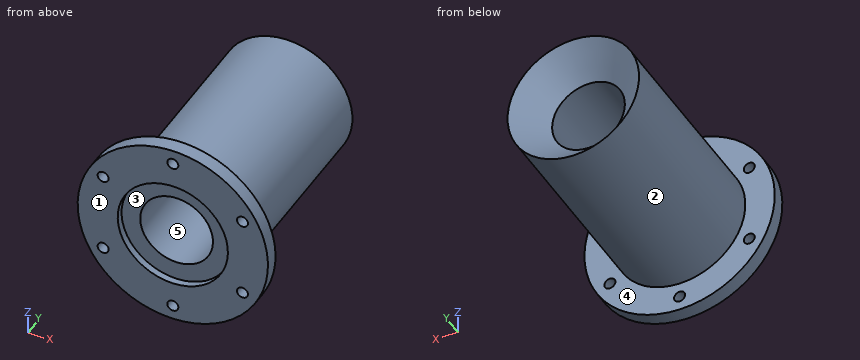
```python
from build123d import *

# Parameters (mm, degrees)
SKETCH_2_R          = 1.5
CUT_EXTRUDE_1_DEPTH = 10


with BuildPart() as part:
    # Эскиз1 → Повернуть1 (revolve)
    with BuildSketch(Plane(origin=(0, 0, 0), x_dir=(0, 0, -1), z_dir=(1, 0, 0))):
        Polygon((9.9, 52), (9.9, 2), (15, 2), (15, 0), (25.9, 0), (25.9, 4), (17.9, 4), (17.9, 60), align=None)
    revolve(axis=Axis((0, 0, 0), (0, 1, 0)))

    # Эскиз2 → Вырез-Вытянуть1 (cut)
    with BuildSketch(Plane(origin=(0, 4, 0), x_dir=(1, 0, 0), z_dir=(0, 1, 0))):
        with Locations(Location((0, 21.9, 0), (0, 0, 270))):
            Circle(SKETCH_2_R)
        with Locations(Location((18.965956343, 10.95, 0), (0, 0, 270))):
            Circle(SKETCH_2_R)
        with Locations(Location((18.965956343, -10.95, 0), (0, 0, 270))):
            Circle(SKETCH_2_R)
        with Locations(Location((0, -21.9, 0), (0, 0, 270))):
            Circle(SKETCH_2_R)
        with Locations(Location((-18.965956343, -10.95, 0), (0, 0, 270))):
            Circle(SKETCH_2_R)
        with Locations(Location((-18.965956343, 10.95, 0), (0, 0, 270))):
            Circle(SKETCH_2_R)
    extrude(amount=-CUT_EXTRUDE_1_DEPTH, mode=Mode.SUBTRACT)


solid = part.part
```
The model under review builds one solid part; all positions refer to its coordinate system, in mm. Face numbers are marked on the shaded views. A direction names the side the tool comes from. Round coordinates to 2 decimals unless told otherwise and drop trailing zeros. Write each loop counter-clockwise with the first axis right and the second up, starting at its lowest first coordinate (ties: lowest second). Pieces come first, ordered by that corner, then holes. Notation, with made-up numbers: M 29.5,-35 L 70.5,-35 A24 ccw 70.5,-25 Z; hole C 20.25,24 d2. An arc over 180 degrees is marked long. Use CSV: the item, a comma, the result in double quotes. Start each with the question number.
(1) For line 1 along Y through (x, z) = (15, 12.5); line 2 along X through (y, z) = (21, 0); line 3 along X through (y, z) = (1.4, 21.9), list the stretches that pass through material, from the lowest coordinate up.
(2) We need section A-A, the plane z = 0. State the section outline as (x, y) points, then the cut area to 3 significant figures.
(3) We need section D-D, the plane z = 21.9. State the section outline as (x, y) points, then the cut area to 3 significant figures.
(4) We need section C-C, the plane y = 53.5. State the section outline as (x, z) points, then the cut area to 3 significant figures.
(5) The part is to be moulded in two halves that separate along Z. For the marked faces 1, 2 and 3, say which applies: +Z half, -Z half, draft (parallel to the pull), parting line (faces both ways), or undercut.
(6) Tool access review of the marked faces 4 and 5: name each direction out of +Z, -Z, +X, -X, +Y, -Y from which nothing blocks a thin tool from reaching the whole face with its end or side.
(7) We need section B-B, the plane x = 0. State the section outline as (y, z) points, then the cut area to 3 significant figures.
(8) Clearance check with flat-ended pins moving along their axes: P1, Ø6, axis at x = -12.5, z = -16, coming from the -Y side; P2, Ø15, axis at x = 5, z = -5, coming from the -Y side; P3, Ø2, axis at x = -6.5, z = -7, coming from the +Y side; P4, Ø6, axis at x = -9.5, y = 8, coming from the +Z side. State where each tip first meets the part, or that it passes through.
Findings:
1,line 1,"0 to 4"
1,line 2,"-17.9 to -9.9, 9.9 to 17.9"
1,line 3,"-13.83 to -1.5, 1.5 to 13.83"
2,outline,"M -25.9,0 L -15,0 L -15,2 L -9.9,2 L -9.9,52 L -17.9,60 L -17.9,4 L -25.9,4 Z; M 9.9,2 L 15,2 L 15,0 L 25.9,0 L 25.9,4 L 17.9,4 L 17.9,60 L 9.9,52 Z"
2,area,"940 mm^2"
3,outline,"M -13.83,0 L -1.5,0 L -1.5,4 L -13.83,4 Z; M 1.5,0 L 13.83,0 L 13.83,4 L 1.5,4 Z"
3,area,"98.6 mm^2"
4,outline,"C 0,0 d35.8; hole C 0,0 d22.8"
4,area,"598 mm^2"
5,face 1,"draft"
5,face 2,"parting line"
5,face 3,"undercut"
6,face 4,"+Y"
6,face 5,"+Y, -Y"
7,outline,"M 0,-25.9 L 4,-25.9 L 4,-23.4 L 0,-23.4 Z; M 0,-20.4 L 4,-20.4 L 4,-17.9 L 60,-17.9 L 52,-9.9 L 2,-9.9 L 2,-15 L 0,-15 Z; M 0,15 L 2,15 L 2,9.9 L 52,9.9 L 60,17.9 L 4,17.9 L 4,20.4 L 0,20.4 Z; M 0,23.4 L 4,23.4 L 4,25.9 L 0,25.9 Z"
7,area,"916 mm^2"
8,P1,"y = 0"
8,P2,"y = 2"
8,P3,"y = 52.65"
8,P4,"z = 16.68"
